```python
from build123d import *
from OCP.BRepFilletAPI import BRepFilletAPI_MakeChamfer

# Parameters (mm, degrees)
SKETCH4_W                = 12.46
SKETCH4_H                = 17.25
BOSS_EXTRUDE3_DEPTH      = 6
BOSS_EXTRUDE6_DEPTH      = 7.3
BOSS_EXTRUDE6_DEPTH_BACK = 17.25
SKETCH8_R                = 12.546781182
SKETCH8_R_2              = 11.15
BOSS_EXTRUDE4_DEPTH      = 17.25
SKETCH6_R                = 2
CUT_EXTRUDE1_DEPTH       = 5
CHAMFER1_SIZE            = 0.5
CHAMFER1_SIZE_2          = 0.866025404
SKETCH10_W               = 12.46
SKETCH10_H               = 23.7
CUT_EXTRUDE3_DEPTH       = 17.25
CUT_EXTRUDE4_REACH       = 43.938
SKETCH11_W               = 5
SKETCH11_H               = 3
BOSS_EXTRUDE7_START      = -7.3
BOSS_EXTRUDE7_DEPTH      = 7.3
BOSS_EXTRUDE9_START      = 10
BOSS_EXTRUDE9_DEPTH      = 10
BOSS_EXTRUDE10_DEPTH     = 34.55
SKETCH18_W               = 20
SKETCH18_H               = 12.438292938
CUT_EXTRUDE5_DEPTH       = 2
CUT_EXTRUDE6_DEPTH       = 58.651133872
CUT_EXTRUDE6_DEPTH_BACK  = 58.651133872
SKETCH19_R               = 1.25
FILLET1_R                = 10


with BuildPart() as part:
    # Sketch4 → Boss-Extrude3 (new body)
    with BuildSketch(Plane.XY):
        with Locations((0, -1.35)):
            Rectangle(SKETCH4_W, SKETCH4_H)
    extrude(amount=BOSS_EXTRUDE3_DEPTH)



with BuildPart() as body_2:
    # Sketch8 → Boss-Extrude6 (new, two sides: drawn at the far end of the back side and taken through both)
    with BuildSketch(Plane(origin=(0, -9.975, 0), x_dir=(-1, 0, 0), z_dir=(0, -1, 0)).offset(-BOSS_EXTRUDE6_DEPTH_BACK)):
        with Locations(Location((0, -23.55, 0), (0, 0, 90))):
            Circle(SKETCH8_R)
        with Locations(Location((0, -23.55, 0), (0, 0, 90))):
            Circle(SKETCH8_R_2, mode=Mode.SUBTRACT)
    extrude(amount=BOSS_EXTRUDE6_DEPTH + BOSS_EXTRUDE6_DEPTH_BACK)


with BuildPart() as part_1:
    add(part.part)

    add(body_2.part)  # Boss-Extrude4 merges body 2
    # Sketch5 → Boss-Extrude4 (add)
    with BuildSketch(Plane(origin=(0, 7.275, 0), x_dir=(1, 0, 0), z_dir=(0, 1, 0))):
        with BuildLine():
            Line((12.546781182, -23.55), (12.546781182, 0))
            Line((12.546781182, 0), (6.23, 0))
            Line((6.23, 0), (6.23, -29.7))
            Line((6.23, -29.7), (-6.23, -29.7))
            Line((-6.23, -29.7), (-6.23, 0))
            Line((-6.23, 0), (-12.546781182, 0))
            Line((-12.546781182, 0), (-12.546781182, -23.55))
            ThreePointArc((-12.546781182, -23.55), (0, -36.096781182), (12.546781182, -23.55))
        make_face()
    extrude(amount=-BOSS_EXTRUDE4_DEPTH)

    # Sketch6 → Cut-Extrude1 (cut)
    with BuildSketch(Plane(origin=(0, 7.275, 0), x_dir=(1, 0, 0), z_dir=(0, 1, 0))):
        with Locations(Location((0, -3.5, 0), (0, 0, 270))):
            Circle(SKETCH6_R)
        with Locations(Location((0, -32.2, 0), (0, 0, 270))):
            Circle(SKETCH6_R)
    extrude(amount=-CUT_EXTRUDE1_DEPTH, mode=Mode.SUBTRACT)

    # Chamfer1
    chamfer1_edges_1 = [part_1.edges().sort_by_distance(p)[0] for p in [
        (0, 7.275, 1.5),
    ]]
    chamfer1_side_1 = [part_1.faces().sort_by_distance(p)[0] for p in [
        (0, 7.275, 1.49),
    ]]
    chamfer1_edges_2 = [part_1.edges().sort_by_distance(p)[0] for p in [
        (0, 7.275, 30.2),
    ]]
    chamfer1_side_2 = [part_1.faces().sort_by_distance(p)[0] for p in [
        (0, 7.275, 30.19),
    ]]
    chamfer1 = BRepFilletAPI_MakeChamfer(part_1.part.solid().wrapped)
    for e in chamfer1_edges_1:
        chamfer1.Add(CHAMFER1_SIZE - 0.0001, CHAMFER1_SIZE_2 - 0.0001, e.wrapped, chamfer1_side_1[0].wrapped)
    for e in chamfer1_edges_2:
        chamfer1.Add(CHAMFER1_SIZE - 0.0001, CHAMFER1_SIZE_2 - 0.0001, e.wrapped, chamfer1_side_2[0].wrapped)
    add(Compound.cast(chamfer1.Shape()), mode=Mode.REPLACE)  # a hair under: the kernel refuses the full size

    # Sketch10 → Cut-Extrude3 (cut)
    with BuildSketch(Plane(origin=(0, 7.275, 0), x_dir=(1, 0, 0), z_dir=(0, 1, 0))):
        with Locations((0, -17.85)):
            Rectangle(SKETCH10_W, SKETCH10_H)
    extrude(amount=-CUT_EXTRUDE3_DEPTH, mode=Mode.SUBTRACT)

    # Sketch11 → Cut-Extrude4 (cut, up to next)
    with BuildSketch(Plane.XY.offset(36.096781182), mode=Mode.PRIVATE) as cut_extrude4_sk1:
        with Locations((0, -8.475)):
            Rectangle(SKETCH11_W, SKETCH11_H)
    cut_extrude4_tool1 = extrude(cut_extrude4_sk1.sketch, amount=-CUT_EXTRUDE4_REACH, mode=Mode.PRIVATE) & part_1.part
    add(cut_extrude4_tool1.solids().sort_by_distance((0, -8.475, 36.096781))[0], mode=Mode.SUBTRACT)

    # Sketch13 → Boss-Extrude7 (add)
    with BuildSketch(Plane.XZ.offset(17.275).offset(BOSS_EXTRUDE7_START)):
        with BuildLine():
            Line((-12.546781182, 23.55), (-12.546781182, 0))
            Line((-12.546781182, 0), (12.546781182, 0))
            Line((12.546781182, 0), (12.546781182, 23.55))
            ThreePointArc((12.546781182, 23.55), (0, 11.003218818), (-12.546781182, 23.55))
        make_face()
    extrude(amount=BOSS_EXTRUDE7_DEPTH)

    # Sketch15 → Boss-Extrude9 (add)
    with BuildSketch(Plane(origin=(0, 7.275, 0), x_dir=(1, 0, 0), z_dir=(0, 1, 0)).offset(BOSS_EXTRUDE9_START)):
        with BuildLine():
            Line((-12.546781182, 0), (12.546781182, 0))
            Line((12.546781182, 0), (12.546781182, -23.55))
            ThreePointArc((12.546781182, -23.55), (0, -36.096781182), (-12.546781182, -23.55))
            Line((-12.546781182, -23.55), (-12.546781182, 0))
        make_face()
        with BuildLine():
            Line((-6.23, -0.8), (6.23, -0.8))
            Line((6.23, -0.8), (6.23, -33.5))
            ThreePointArc((6.23, -33.5), (5.937106781, -34.207106781), (5.23, -34.5))
            Line((5.23, -34.5), (-5.23, -34.5))
            ThreePointArc((-5.23, -34.5), (-5.937106781, -34.207106781), (-6.23, -33.5))
            Line((-6.23, -33.5), (-6.23, -0.8))
        make_face(mode=Mode.SUBTRACT)
    extrude(amount=-BOSS_EXTRUDE9_DEPTH)

    # Sketch17 → Boss-Extrude10 (add)
    with BuildSketch(Plane(origin=(0, 17.275, 0), x_dir=(1, 0, 0), z_dir=(0, 1, 0))):
        Polygon((21.75, 25), (21.75, 0), (-21.75, 0), (-21.75, 25), (-17.75, 25), (-17.75, 5), (17.75, 5), (17.75, 25), align=None)
    extrude(amount=-BOSS_EXTRUDE10_DEPTH)

    # Sketch18 → Cut-Extrude5 (cut)
    with BuildSketch(Plane.ZY.offset(-17.75)):
        with Locations((-15, 0)):
            Rectangle(SKETCH18_W, SKETCH18_H)
    extrude(amount=-CUT_EXTRUDE5_DEPTH, mode=Mode.SUBTRACT)

    # Sketch19 → Cut-Extrude6 (cut, two sides: drawn at the far end of the back side and taken through both)
    with BuildSketch(Plane.ZY.offset(-19.75).offset(-CUT_EXTRUDE6_DEPTH_BACK)):
        with Locations((-20, 0)):
            Circle(SKETCH19_R)
    extrude(amount=CUT_EXTRUDE6_DEPTH + CUT_EXTRUDE6_DEPTH_BACK, mode=Mode.SUBTRACT)

    # Fillet1
    fillet1_edges = [part_1.edges().sort_by_distance(p)[0] for p in [
        (19.75, 17.275, -25),
        (-19.75, 17.275, -25),
        (-19.75, -17.275, -25),
        (19.75, -17.275, -25),
    ]]
    fillet(fillet1_edges, radius=FILLET1_R)


solid = part_1.part
```
Model file for the job. Use its own axes, mm. A direction names the side the tool comes from. Coordinates: 2 decimals unless noted, no trailing zeros. Loops run counter-clockwise (first coordinate to the right, second up) from the corner with the lowest first, then second, coordinate; pieces in that order, holes last. Notation, with made-up numbers: (19, -37) -> (24, -37) arc R26 cw to (24, -19) -> close; hole circle Ø1 at (-1.75, 49.5). An arc over 180 degrees is marked (long way). Answer as a JSON object with one key per item and string values.
Q1. Cut at D-D (y = 9). List the corners of the cut face in (x, z).
Report:
{"outline": "(-21.75, -24.85) -> (-17.75, -24.85) -> (-17.75, -5) -> (17.75, -5) -> (17.75, -24.85) -> (21.75, -24.85) -> (21.75, 0) -> (12.55, 0) -> (12.55, 23.55) arc R12.55 ccw to (-12.55, 23.55) -> (-12.55, 0) -> (-21.75, 0) -> close; hole (-6.23, 0.8) -> (6.23, 0.8) -> (6.23, 33.5) arc R1 ccw to (5.23, 34.5) -> (-5.23, 34.5) arc R1 ccw to (-6.23, 33.5) -> close"}
Q2. Probe probe 1 along X at (y, z) = (15, 24); probe 2 along Z at (x, y) = (-19.55, 0); probe 3 along X at (y, z) = (-13, -20.5). List the from-to ranges inside material, lowest first.
Report:
{"probe 1": "x = -12.54 to -6.23, 6.23 to 12.54", "probe 2": "z = -25 to -21.25, -18.75 to 0", "probe 3": "x = -21.75 to -17.75, 17.75 to 21.75"}
Q3. Cut at B-B (x = 0). State how many separate pieces and enclosed holes the cut face has, and give its area (3 significant figures).
Report:
{"separate pieces": "3", "enclosed holes": "0", "area": "451 mm2"}
Q4. Pull direction X, two halves, no side cores. Call faces 1 (the cylindrical face through (19.778, 14.268, -22.148)), 2 (the cylindrical face through (0.276, 0.242, 36.094)), 3 (the flat face through (12.547, 0, 12)), 4 (the flat face through (19.75, 0, -15)): released by +X, released by -X, zero draft, split by the parting line, or undercut.
Report:
{"face 1": "zero draft", "face 2": "split by the parting line", "face 3": "released by +X", "face 4": "undercut"}
Q5. Cut at C-C (z = 26). List the corners of the cut face in (x, y) (1 decimal).
Report:
{"outline": "(-12.3, -17.3) -> (-10.9, -17.3) -> (-10.9, -10) -> (-6.2, -10) -> (-6.2, 17.3) -> (-12.3, 17.3) -> close; (6.2, -10) -> (10.9, -10) -> (10.9, -17.3) -> (12.3, -17.3) -> (12.3, 17.3) -> (6.2, 17.3) -> close"}
Q6. Cut at A-A (y = 0). List the corners of the cut face in (x, z).
Report:
{"outline": "(-21.75, -25) -> (-17.75, -25) -> (-17.75, -21.25) -> (-21.75, -21.25) -> close; (-21.75, -18.75) -> (-17.75, -18.75) -> (-17.75, -5) -> (19.75, -5) -> (19.75, -18.75) -> (21.75, -18.75) -> (21.75, 0) -> (12.55, 0) -> (12.55, 23.55) arc R12.55 ccw to (-12.55, 23.55) -> (-12.55, 0) -> (-21.75, 0) -> close; (19.75, -25) -> (21.75, -25) -> (21.75, -21.25) -> (19.75, -21.25) -> close; hole (-6.23, 6) -> (6.23, 6) -> (6.23, 29.7) -> (-6.23, 29.7) -> close"}
Q7. Flat gauge pins, fed straight in: P1, Ø12, axis at x = 5, y = -13, coming from the -Z side; P2, Ø6, axis at y = 3.5, z = 16.5, coming from the -X side; P3, Ø3.5, axis at x = -2, y = 0, coming from the +Z side; P4, Ø4, axis at x = 0.5, z = 26.5, coming from the +Y side. Where does each tip first touch, or does it go through?
Report:
{"P1": "stops at z = -5", "P2": "stops at x = -12.55", "P3": "stops at z = 36.09", "P4": "passes through"}
Q8. 3-axis set-ups, long thin cutter, end or side, ignore diameter. For faces 5 (the cylindrical face through (-0.766, 4.371, 34.047)), 6 (the flat face through (-17.75, 0, -15)), 7 (the flat face through (19, 6.219, -15)), 8 (the flat face through (2.5, -8, 33)), 9 (the flat face through (-8, -9.975, 24)): which of +Z, -Z, +X, -X, +Y, -Y reach the whole face in a straight line?
Report:
{"face 5": "+Y", "face 6": "-Z, +Y, -Y", "face 7": "-Z", "face 8": "+Z", "face 9": "-Y"}
